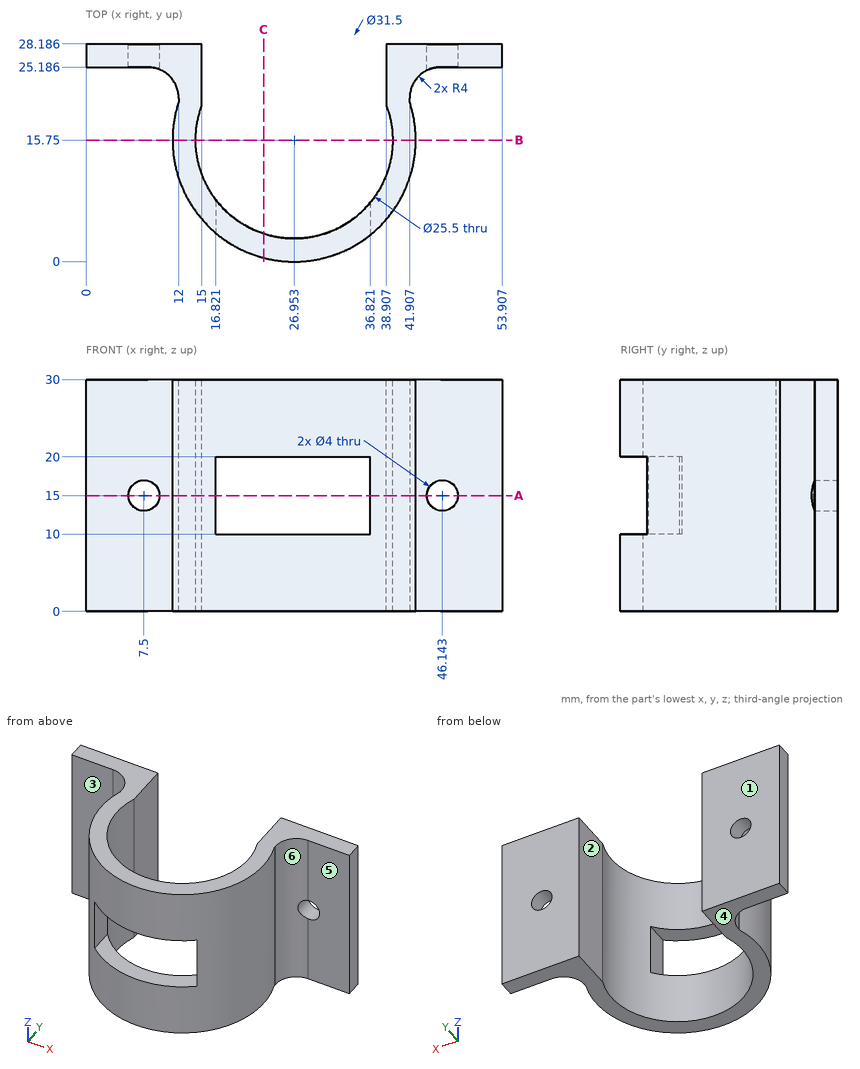
Can you work these out from the drawing? Everything is in mm from the part's minimum corner. A direction names the side the tool comes from. Round coordinates to 2 decimals unless told otherwise and drop trailing zeros. Loops run counter-clockwise (first coordinate to the right, second up) from the corner with the lowest first, then second, coordinate; pieces in that order, holes last. Notation, with made-up numbers: (5, 47.5) -> (46, 47.5) arc R17 ccw to (46, 80.5) -> close; hole circle Ø11 at (-1.5, 66.5). An arc over 180 degrees is marked (long way). Put each result on its own line as item: value.
Q1. I want a section at C-C on x = 23. Write out the boundary of the cut face in (y, z) (1 decimal).
Checks:
outline: (0.5, 0) -> (3.6, 0) -> (3.6, 10) -> (0.5, 10) -> close; (0.5, 20) -> (3.6, 20) -> (3.6, 30) -> (0.5, 30) -> close
Q2. Please list where these lines run through material, in increasing order: line 1 (Z direction, x = 7.5, y = 26.9); line 2 (Z direction, x = 17, y = 5.25); line 3 (X direction, y = 20.75, z = 27.5). Write a range as from..to.
Checks:
line 1: 0..13, 17..30
line 2: 0..10, 20..30
line 3: 12..15, 38.91..41.91
Q3. Thinking about a two-plate mould opening in Y: for the marked faces 4, 5 and 6, which applies, pulls with the +Y half, pulls with the -Y half, needs draft (parallel to the pull), parting line crosses it, or undercut?
Checks:
face 4: needs draft
face 5: pulls with the -Y half
face 6: undercut
Q4. For pin 1 Ø3.5 at (y, z) = (5.5, 15.5) entering from +X; pin 2 Ø3.5 at (y, z) = (5, 16) entering from -X; pin 3 Ø4.5 at (x, z) = (46.14, 15) entering from -Y; pin 4 Ø3 at (x, z) = (7.5, 15) entering from +Y, each with a flat end and sliding along its axis, tell me the tip position at first contact or that it passes through.
Checks:
pin 1: x = 40.21
pin 2: x = 14.03
pin 3: y = 24.64
pin 4: through
Q5. I want a section at B-B on y = 15.75. Write out the boundary of the cut face in (x, z), and give its area (3 significant figures).
Checks:
outline: (11.2, 0) -> (14.2, 0) -> (14.2, 30) -> (11.2, 30) -> close; (39.7, 0) -> (42.7, 0) -> (42.7, 30) -> (39.7, 30) -> close
area: 180 mm2
Q6. I want a section at A-A on z = 15. Give the number of separate pieces and of enclosed holes in the cut face, and give its area (3 significant figures).
Checks:
separate pieces: 4
enclosed holes: 0
area: 197 mm2
Q7. Which directions (+Z, -Z, +X, -X, +Y, -Y) give clear straight access to the entire face, cutting with the end or side of a thin tool? Please do the marked faces 1, 2 and 3.
Checks:
face 1: +Z, -Z, +X, -X, +Y
face 2: +Z, -Z, +Y
face 3: +Z, -Z, -X, -Y
